For this review, take the finished solid that the model builds, in its own axes (mm). A direction names the side the tool comes from. Coordinates: 2 decimals unless noted, no trailing zeros. Order: outer loops, then holes, each group sorted by start corner. A loop starts at its lowest first (then second) coordinate and runs counter-clockwise, first axis right, second up.
from build123d import *

# Parameters (mm, degrees)
SKETCH2_R          = 1.5
CUT_EXTRUDE1_DEPTH = 4.95


with BuildPart() as part:
    # Sketch1 → Revolve1 (revolve)
    with BuildSketch(Plane.XY):
        Polygon((12, 0), (12, -1.6), (5, -1.6), (5, -3.95), (3, -3.95), (3, 0), align=None)
    revolve(axis=Axis((0, 0, 0), (0, 1, 0)))

    # Sketch2 → Cut-Extrude1 (cut, through all)
    with BuildSketch(Plane(origin=(0, 0, 0), x_dir=(1, 0, 0), z_dir=(0, 1, 0))):
        with Locations((8.4, 0)):
            Circle(SKETCH2_R)
        with Locations((-8.4, 0)):
            Circle(SKETCH2_R)
    extrude(amount=-CUT_EXTRUDE1_DEPTH, mode=Mode.SUBTRACT)


solid = part.part
1. The part is to be moulded in two halves that separate along Z. For faces 3 (the face through (-2.5, 0, 2.5)), 4 (the face through (-3, -2, 0)), 5 (the face through (-1.08, -2.79, 4.88)), say which applies: +Z half, -Z half, draft (parallel to the pull), parting line (faces both ways), or undercut.
Answer below:
face 3: draft
face 4: undercut
face 5: parting line
2. Take a section at D-D, the plane z = -3.5. Give the boundary of the cut face in (x, y).
Answer below:
outline: (-11.48, -1.6) - (-3.57, -1.6) - (-3.57, -3.95) - (3.57, -3.95) - (3.57, -1.6) - (11.48, -1.6) - (11.48, 0) - (-11.48, 0) - close
3. Take a section at A-A, the plane x = 0. Give the boundary of the cut face in (y, z).
Answer below:
outline: (-3.95, -5) - (-1.6, -5) - (-1.6, -12) - (0, -12) - (0, -3) - (-3.95, -3) - close; (-3.95, 3) - (0, 3) - (0, 12) - (-1.6, 12) - (-1.6, 5) - (-3.95, 5) - close
4. Take a section at B-B, the plane z = 0. Give the boundary of the cut face in (x, y), plus the area to 3 significant figures.
Answer below:
outline: (-12, -1.6) - (-9.9, -1.6) - (-9.9, 0) - (-12, 0) - close; (-6.9, -1.6) - (-5, -1.6) - (-5, -3.95) - (-3, -3.95) - (-3, 0) - (-6.9, 0) - close; (3, -3.95) - (5, -3.95) - (5, -1.6) - (6.9, -1.6) - (6.9, 0) - (3, 0) - close; (9.9, -1.6) - (12, -1.6) - (12, 0) - (9.9, 0) - close
area: 28.6 mm2
5. Take a section at C-C, the plane y = -3.05. Give the boundary of the cut face in (x, z).
Answer below:
outline: circle Ø10 at (0, 0); hole circle Ø6 at (0, 0)
6. Machinability: for faces 1 (the face through (5.2, -1.6, -0.2)), 2 (the face through (7.2, -0.8, 0.9)), which of the approach directions +Z, -Z, +X, -X, +Y, -Y give a long, thin tool a straight path to every point of the face, cutting with its end or side? Answer none if there is none.
Answer below:
face 1: -Y
face 2: +Y, -Y
7. Clearance check with flat-ended pins moving along their axes: pin 1 Ø4 at (x, z) = (8.4, 0) entering from -Y; pin 2 Ø1.5 at (x, y) = (3.5, -1.5) entering from +Z; pin 3 Ø3.5 at (x, z) = (0, 0) entering from +Y. State where each tip first meets the part, or that it passes through.
Answer below:
pin 1: stops at y = -1.6
pin 2: stops at z = 11.68
pin 3: passes through
8. To check wall thickness, follow L1, parallel to X at y = -0.5, z = 0; L2, parallel to Y at x = 7.5, z = 6; L3, parallel to Z at x = -8.4, y = -0.5. State the ranges of each line that lie inside material, in increasing order.
Answer below:
L1: x = -12 to -9.9, -6.9 to -3, 3 to 6.9, 9.9 to 12
L2: y = -1.6 to 0
L3: z = -8.57 to -1.5, 1.5 to 8.57
